```python
from build123d import *

# Parameters (mm, degrees)
SKETCH1_W           = 85
SKETCH1_H           = 14
BOSS_EXTRUDE1_DEPTH = 2
SKETCH2_W           = 85
SKETCH2_H           = 2
BOSS_EXTRUDE2_DEPTH = 6
CUT_EXTRUDE1_DEPTH  = 4
SKETCH4_W           = 10
SKETCH4_H           = 10
BOSS_EXTRUDE3_DEPTH = 2
CUT_EXTRUDE2_DEPTH  = 20
CHAMFER1_SIZE       = 1.5
SKETCH6_W           = 10
SKETCH6_H           = 10
BOSS_EXTRUDE4_DEPTH = 50
CUT_EXTRUDE3_DEPTH  = 50
FILLET1_R           = 10
CUT_EXTRUDE4_DEPTH  = 10


with BuildPart() as part:
    # Sketch1 → Boss-Extrude1 (new body)
    with BuildSketch(Plane.XY):
        with Locations((-9.558823529, 4.906862745)):
            Rectangle(SKETCH1_W, SKETCH1_H)
    extrude(amount=BOSS_EXTRUDE1_DEPTH)

    # Sketch2 → Boss-Extrude2 (add)
    with BuildSketch(Plane.XY):
        with Locations((-9.558823529, -1.093137255)):
            Rectangle(SKETCH2_W, SKETCH2_H)
    extrude(amount=BOSS_EXTRUDE2_DEPTH)

    # Sketch3 → Cut-Extrude1 (cut)
    with BuildSketch(Plane.XY.offset(6)):
        Polygon((32.941176471, -0.093137255), (7.941176471, -0.093137255), (12.941176471, -2.093137255), (32.941176471, -2.093137255), align=None)
    extrude(amount=-CUT_EXTRUDE1_DEPTH, mode=Mode.SUBTRACT)

    # Sketch4 → Boss-Extrude3 (add)
    with BuildSketch(Plane(origin=(0, 0, 0), x_dir=(-1, 0, 0), z_dir=(0, 0, -1))):
        with Locations((-37.941176471, 6.906862745)):
            Rectangle(SKETCH4_W, SKETCH4_H)
    extrude(amount=-BOSS_EXTRUDE3_DEPTH)

    # Sketch5 → Cut-Extrude2 (cut)
    with BuildSketch(Plane.XZ.offset(2.093137255)):
        Polygon((-52.058823529, 0), (-36.428289141, 6), (-52.058823529, 6), align=None)
    extrude(amount=-CUT_EXTRUDE2_DEPTH, mode=Mode.SUBTRACT)

    # Chamfer1
    chamfer1_edges = [part.edges().sort_by_distance(p)[0] for p in [
        (-44.243556335, -2.093137255, 3),
    ]]
    chamfer(chamfer1_edges, length=CHAMFER1_SIZE)

    # Sketch6 → Boss-Extrude4 (add)
    with BuildSketch(Plane(origin=(42.941176471, 0, 0), x_dir=(0, 0, -1), z_dir=(1, 0, 0))):
        with Locations((-7, 6.906862745)):
            Rectangle(SKETCH6_W, SKETCH6_H)
    extrude(amount=-BOSS_EXTRUDE4_DEPTH)

    # Sketch7 → Cut-Extrude3 (cut)
    with BuildSketch(Plane.XZ.offset(-1.906862745)):
        Polygon((42.941176471, 0), (38.092861761, 12), (42.941176471, 12), align=None)
    extrude(amount=-CUT_EXTRUDE3_DEPTH, mode=Mode.SUBTRACT)

    # Fillet1
    fillet1_edges = [part.edges().sort_by_distance(p)[0] for p in [
        (40.517019116, 11.906862745, 6),
    ]]
    fillet(fillet1_edges, radius=FILLET1_R - 0.0001)  # a hair under: the kernel refuses the full size

    # Sketch8 → Cut-Extrude4 (cut)
    with BuildSketch(Plane.XY.offset(12)):
        with BuildLine():
            Line((-7.058823529, 11.906862745), (-7.058823529, 1.906862745))
            Line((-7.058823529, 1.906862745), (38.092861761, 1.906862745))
            add(Edge.make_bspline(
                [(-7.058823529, 11.906862745), (7.597424673, 10.416193164), (26.985171478, 14.416758063), (38.092861761, 1.906862745)],
                knots=[0, 0, 0, 0, 1, 1, 1, 1], degree=3))
        make_face()
    extrude(amount=-CUT_EXTRUDE4_DEPTH, mode=Mode.SUBTRACT)


solid = part.part
```
The model under review builds one solid part; all positions refer to its coordinate system, in mm. A direction names the side the tool comes from. Round coordinates to 2 decimals unless told otherwise and drop trailing zeros. Loops run counter-clockwise (first coordinate to the right, second up) from the corner with the lowest first, then second, coordinate; pieces in that order, holes last.
1) Clearance check with flat-ended pins moving along their axes: P1, Ø1.6, axis at x = -2, y = -1, coming from the +Z side; P2, Ø1, axis at y = -0.5, z = 1, coming from the +X side. State where each tip first meets the part, or that it passes through.
Values follow:
P1: stops at z = 6
P2: stops at x = 32.94
2) Wall thickness on line 1 along Y through (x, z) = (-35.5, 2.5); line 2 along Z through (x, y) = (-31, 7.75); line 3 along Z through (x, y) = (7.5, -1): over which ranges is each line inside the solid? List them lowest first.
Values follow:
line 1: y = -2.09 to -0.09
line 2: z = 0 to 2
line 3: z = 0 to 6
3) Consider section A-A on x = -13.5. State the section outline as (y, z) points.
Values follow:
outline: (-2.09, 0) - (11.91, 0) - (11.91, 2) - (-0.09, 2) - (-0.09, 6) - (-2.09, 6) - close
4) Tool access review of faces 1 (the face through (-20, -0.093, 4)), 2 (the face through (39, 1.907, 3)), 3 (the face through (-12, -1, 6)), 4 (the face through (10.41, -1.08, 4.03)): name each direction out of +Z, -Z, +X, -X, +Y, -Y from which nothing blocks a thin tool from reaching the whole face with its end or side.
Values follow:
face 1: +Z, +X, -X
face 2: +Z, -Z, +X, -Y
face 3: +Z, +X, -X, -Y
face 4: +Z, +X
5) Consider section B-B on x = -45. State the section outline as (y, z) points.
Values follow:
outline: (-2.09, 0) - (11.91, 0) - (11.91, 2) - (-0.09, 2) - (-0.09, 2.71) - (-0.59, 2.71) - (-2.09, 1.1) - close
